```python
from build123d import *

# Parameters (mm, degrees)
SKETCH1_W           = 23
SKETCH1_H           = 11
BOSS_EXTRUDE1_DEPTH = 16
SKETCH2_W           = 32
SKETCH2_H           = 11
BOSS_EXTRUDE2_DEPTH = 2.5
SKETCH3_W           = 23
SKETCH3_H           = 11
BOSS_EXTRUDE3_DEPTH = 5
BOSS_EXTRUDE4_DEPTH = 5
BOSS_EXTRUDE5_DEPTH = 3


with BuildPart() as part:
    # Sketch1 → Boss-Extrude1 (new body)
    with BuildSketch(Plane(origin=(0, 0, 0), x_dir=(1, 0, 0), z_dir=(0, 1, 0))):
        Rectangle(SKETCH1_W, SKETCH1_H)
    extrude(amount=BOSS_EXTRUDE1_DEPTH)

    # Sketch2 → Boss-Extrude2 (add)
    with BuildSketch(Plane(origin=(0, 16, 0), x_dir=(1, 0, 0), z_dir=(0, 1, 0))):
        Rectangle(SKETCH2_W, SKETCH2_H)
    extrude(amount=BOSS_EXTRUDE2_DEPTH)

    # Sketch3 → Boss-Extrude3 (add)
    with BuildSketch(Plane(origin=(0, 18.5, 0), x_dir=(1, 0, 0), z_dir=(0, 1, 0))):
        Rectangle(SKETCH3_W, SKETCH3_H)
    extrude(amount=BOSS_EXTRUDE3_DEPTH)

    # Sketch4 → Boss-Extrude4 (add)
    with BuildSketch(Plane(origin=(0, 23.5, 0), x_dir=(1, 0, 0), z_dir=(0, 1, 0))):
        with BuildLine():
            ThreePointArc((11.5, 0), (2.110912703, 3.889087297), (6, -5.5))
            Line((6, -5.5), (6, 0))
            Line((6, 0), (11.5, 0))
        make_face()
        with BuildLine():
            Line((6, 0), (6, -5.5))
            ThreePointArc((6, -5.5), (9.889087297, -3.889087297), (11.5, 0))
            Line((11.5, 0), (6, 0))
        make_face()
    extrude(amount=BOSS_EXTRUDE4_DEPTH)

    # Sketch5 → Boss-Extrude5 (add)
    with BuildSketch(Plane(origin=(0, 28.5, 0), x_dir=(1, 0, 0), z_dir=(0, 1, 0))):
        with BuildLine():
            ThreePointArc((8, 0), (4.585786438, 1.414213562), (6, -2))
            Line((6, -2), (6, 0))
            Line((6, 0), (8, 0))
        make_face()
        with BuildLine():
            Line((6, 0), (6, -2))
            ThreePointArc((6, -2), (7.414213562, -1.414213562), (8, 0))
            Line((8, 0), (6, 0))
        make_face()
    extrude(amount=BOSS_EXTRUDE5_DEPTH)


solid = part.part
```
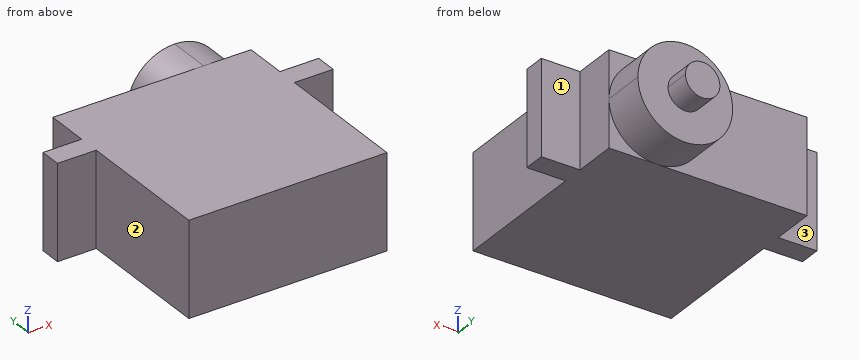
Geometry check sheet. Reference: the model listing, model coordinates, mm. Face numbers are marked on the shaded views. A direction names the side the tool comes from. Give positions to 0.01 mm unless a question says otherwise; leave off trailing zeros. Order: outer loops, then holes, each group sorted by start corner. A loop starts at its lowest first (then second) coordinate and runs counter-clockwise, first axis right, second up. Notation, with made-up numbers: (-29.75, 26.25) - (-7.75, 26.25) arc R28 ccw to (-7.75, 59.25) - close; hole circle Ø6 at (7, 41). An arc over 180 degrees is marked (long way). Write item = value, one per line. Start each with the question number.
1) Access from +Z, -Z, +X, -X, +Y, -Y to the whole of each face (thin tool, end or side, straight path). Record for the marked faces 1, 2 and 3.
2) Section check C-C (y = 2). Enter the section's corners in (x, z).
3) Gauge pin test, flat ends, axial feed: pin 1 Ø4 at (y, z) = (20, 2) entering from +X; pin 2 Ø2 at (x, z) = (-13.5, 2) entering from +Y; pin 3 Ø3 at (x, z) = (9.5, 3.5) entering from +Y; pin 4 Ø3.5 at (y, z) = (4, -1.5) entering from +X. Record the tip position at first contact, or that the pin passes through.
4) Section check D-D (z = -2.5). Enter the section's corners in (x, y).
5) Section check A-A (x = -12.5). Enter the section's corners in (y, z).
6) Scan lines: L1, parallel to Y at x = 13, z = -3.25; L2, parallel to Y at x = 2.5, z = -0.75; L3, parallel to X at y = 4, z = 4.75. Record each from-to range of solid material in increasing order.
Geometry check:
q1.face_1 = +Z, -Z, +X, +Y
q1.face_2 = +Z, -Z, -X, -Y
q1.face_3 = +Z, -Z, -X, +Y
q2.outline = (-11.5, -5.5) - (11.5, -5.5) - (11.5, 5.5) - (-11.5, 5.5) - close
q3.pin_1 = 16
q3.pin_2 = 18.5
q3.pin_3 = 28.5
q3.pin_4 = 11.5
q4.outline = (-16, 16) - (-11.5, 16) - (-11.5, 0) - (11.5, 0) - (11.5, 16) - (16, 16) - (16, 18.5) - (11.5, 18.5) - (11.5, 23.5) - (10.9, 23.5) - (10.9, 28.5) - (1.1, 28.5) - (1.1, 23.5) - (-11.5, 23.5) - (-11.5, 18.5) - (-16, 18.5) - close
q5.outline = (16, -5.5) - (18.5, -5.5) - (18.5, 5.5) - (16, 5.5) - close
q6.L1 = 16 to 18.5
q6.L2 = 0 to 28.5
q6.L3 = -11.5 to 11.5
